Part model, mm, in its own coordinate system. Face numbers are marked on the shaded views. Round coordinates to 2 decimals unless told otherwise and drop trailing zeros. Loops run counter-clockwise (first coordinate to the right, second up) from the corner with the lowest first, then second, coordinate; pieces in that order, holes last. Notation, with made-up numbers: (65.5, 82) - (103.5, 82) arc R15 ccw to (103.5, 107) - close; hole circle Ø6 at (60.5, 53). An arc over 180 degrees is marked (long way). Put each result on its own line as item: value.
Autodesk Inventor part; units mm, degrees
ref_plane "YZ Plane" through (0, 0, 0) normal (1, 0, 0) x (0, 1, 0)
ref_plane "XZ Plane" through (0, 0, 0) normal (0, 1, 0) x (-1, 0, 0)
ref_plane "XY Plane" through (0, 0, 0) normal (0, 0, 1) x (1, 0, 0)
sketch "Sketch2" plane through (0, 0, 0) normal (0, 1, 0) x (-1, 0, 0)
  line L0 (3, -13.1703) -> (3, 0)
  line L1 (-7.9775, -27.9) -> (-4.5, -27.9)
  line L2 (-4.5, -27.9) -> (-4.5, -31.1)
  line L3 (-4.5, -31.1) -> (-7.5657, -31.1)
  circle A0 centre (0, -28.5) radius 1.6
  line L4 (-5, -19.8397) -> (-5, 0)
  arc A1 (-6.2857, -23.5513) -> (-7.9775, -27.9) centre (0, -28.5) ccw
  arc A2 (-7.5657, -31.1) -> (6.4615, -23.7832) centre (0, -28.5) ccw
  line L5 (62.6119, 0) -> (-52.77, 0)
  arc A3 (3, -13.1703) -> (6.4615, -23.7832) centre (21, -13.1703) ccw
  line L6 (3, 0) -> (-5, 0)
  arc A4 (-6.2857, -23.5513) -> (-5, -19.8397) centre (-11, -19.8397) ccw
  point P0 (0, 0)
  point P1 (0, 0)
  point P2 (-5, -22.255)
  point P3 (3, -21.0838)
  dimension "d3" = 0.6
  dimension "d4" = 3.2
  dimension "d5" = 3.2
  dimension "d6" = 4.5
  dimension "d8" = 57
  dimension "d9" = 3
  dimension "d10" = 5
  dimension "d11" = 8
  dimension "d12" = 18
  dimension "d15" = 6
extrude "Extrusion1" add sketch "Sketch2" along normal blind 4.5
mirror "Mirror1" about plane through (0, 0, 0) normal (0, 0, 1) of "Extrusion1"
properties part number "Spacer2"
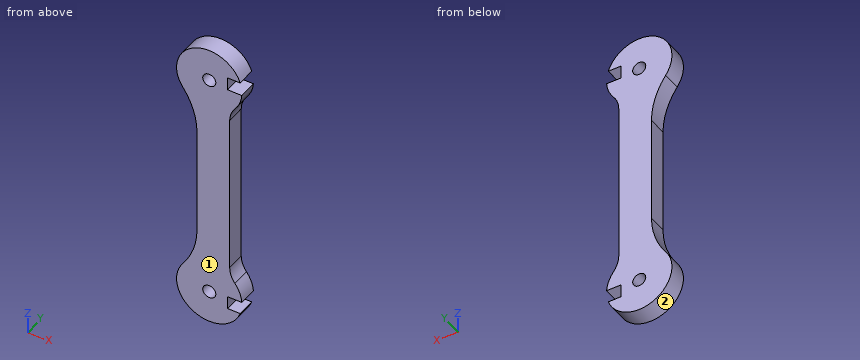
1. Band-saw the part on A-A (x = 0). List the corners of the cut face in (y, z).
A:
outline: (0, -36.5) - (4.5, -36.5) - (4.5, -30.1) - (0, -30.1) - close; (0, -26.9) - (4.5, -26.9) - (4.5, 26.9) - (0, 26.9) - close; (0, 30.1) - (4.5, 30.1) - (4.5, 36.5) - (0, 36.5) - close
2. Band-saw the part on C-C (y = 2.15). List the corners of the cut face in (x, z).
A:
outline: (-6.46, -23.78) arc R8 ccw (long way) to (7.57, -31.1) - (4.5, -31.1) - (4.5, -27.9) - (7.98, -27.9) arc R8 ccw to (6.29, -23.55) arc R6 cw to (5, -19.84) - (5, 19.84) arc R6 cw to (6.29, 23.55) arc R8 ccw to (7.98, 27.9) - (4.5, 27.9) - (4.5, 31.1) - (7.57, 31.1) arc R8 ccw (long way) to (-6.46, 23.78) arc R18 cw to (-3, 13.17) - (-3, -13.17) arc R18 cw to start; hole circle Ø3.2 at (0, -28.5); hole circle Ø3.2 at (0, 28.5)
3. Pin check, flat tips, straight feed: P1, Ø2, axis at x = -5, y = 0.5, coming from the +Z side; P2, Ø1.5, axis at x = 6.5, y = 3, coming from the -Z side; P3, Ø1.5, axis at y = 2.5, z = 1.5, coming from the -X side. Stop position of each tip, or through.
A:
P1: stops at z = 35.43
P2: stops at z = -34.06
P3: stops at x = -3
4. Probe line 1 along Z through (x, y) = (0, 2.5); line 2 along X through (y, z) = (2.25, 28.5); line 3 along Z through (x, y) = (5.75, 2.8). List the from-to ranges inside material, lowest first. Write a range as [from, to].
A:
line 1: z = [-36.5, -30.1], [-26.9, 26.9], [30.1, 36.5]
line 2: x = [-8, -1.6], [1.6, 4.5]
line 3: z = [-34.06, -31.1], [-27.9, -22.74], [22.74, 27.9], [31.1, 34.06]
5. Two-plate mould, pull along Z, no slides. Class the marked faces 1 and 2: pulls with the +Z half, pulls with the -Z half, needs draft (parallel to the pull), parting line crosses it, or undercut.
A:
face 1: needs draft
face 2: undercut
6. Band-saw the part on D-D (x = -4.25). List the corners of the cut face in (y, z), plus the area to 3 significant figures.
A:
outline: (0, -35.28) - (4.5, -35.28) - (4.5, -19.76) - (0, -19.76) - close; (0, 19.76) - (4.5, 19.76) - (4.5, 35.28) - (0, 35.28) - close
area: 140 mm²
7. Band-saw the part on B-B (z = 28.5). List the corners of the cut face in (x, y).
A:
outline: (-8, 0) - (-1.6, 0) - (-1.6, 4.5) - (-8, 4.5) - close; (1.6, 0) - (4.5, 0) - (4.5, 4.5) - (1.6, 4.5) - close
